Autodesk Inventor part; units mm, degrees
ref_plane "YZ Plane" through (0, 0, 0) normal (1, 0, 0) x (0, 1, 0)
ref_plane "XZ Plane" through (0, 0, 0) normal (0, 1, 0) x (-1, 0, 0)
ref_plane "XY Plane" through (0, 0, 0) normal (0, 0, 1) x (1, 0, 0)
sketch "Sketch1" plane through (0, 0, 0) normal (0, 0, 1) x (1, 0, 0)
  line L0 (0, 30.9017) -> (29.3893, 9.5492)
  line L1 (29.3893, 9.5492) -> (18.1636, -25)
  line L2 (18.1636, -25) -> (-18.1636, -25)
  line L3 (-18.1636, -25) -> (-29.3893, 9.5492)
  line L4 (-29.3893, 9.5492) -> (0, 30.9017)
  point P0 (0, 0)
  point P1 (0, 0)
  dimension "d0" = 25
extrude "Extrusion1" add sketch "Sketch1" along normal blind 2 draft 22
properties part number "Face" material "Gold"
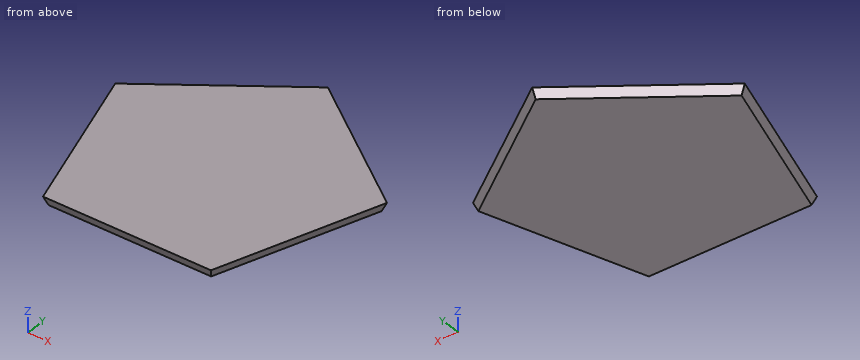
Geometry check sheet. Reference: the model listing, model coordinates, mm. Coordinates: 2 decimals unless noted, no trailing zeros. Loops run counter-clockwise (first coordinate to the right, second up) from the corner with the lowest first, then second, coordinate; pieces in that order, holes last.
Item 1: Sectioned sample at C-C, the plane y = -11. Record the boundary of the cut face in (x, z), then the cut area to 3 significant figures.
Item 2: Sectioned sample at A-A, the plane z = 0.7. Record the boundary of the cut face in (x, y), then the cut area to 3 significant figures.
Item 3: Sectioned sample at B-B, the plane x = 17. Record the boundary of the cut face in (y, z), then the cut area to 3 significant figures.
Item 4: Thickness scan on line 1 (X direction, y = -9, z = 1.05); line 2 (X direction, y = -2.5, z = 1.95); line 3 (Y direction, x = 2, z = 0.7). Record the ranges inside material, lowest first.
Item 5: Go/stop test with a flat-tipped pin: pin 1 Ø1 at (y, z) = (-10.5, 1.5) entering from +X. Record where the tip stops, or that it passes through.
Check result:
1. outline: (-23.56, 2) - (-22.71, 0) - (22.71, 0) - (23.56, 2) - close
1. area: 92.5 mm2
2. outline: (-29.72, 9.66) - (-18.37, -25.28) - (18.37, -25.28) - (29.72, 9.66) - (0, 31.25) - close
2. area: 2,320 mm2
3. outline: (-25.81, 2) - (-25, 0) - (18.55, 0) - (19.55, 2) - close
3. area: 88.9 mm2
4. line 1: x = -23.81 to 23.81
4. line 2: x = -26.3 to 26.3
4. line 3: y = -25.28 to 29.8
5. pin 1: stops at x = 23.78
